```python
from build123d import *

# Parameters (mm, degrees)
SKETCH1_R           = 20.32
BOSS_EXTRUDE1_DEPTH = 26.0985
SKETCH2_W           = 14.0462
SKETCH2_H           = 14.0462
BOSS_EXTRUDE2_DEPTH = 7.7978
SKETCH3_R           = 4.953
BOSS_EXTRUDE3_DEPTH = 10.4013


with BuildPart() as part:
    # Sketch1 → Boss-Extrude1 (new body)
    with BuildSketch(Plane(origin=(0, 0, 0), x_dir=(1, 0, 0), z_dir=(0, 1, 0))):
        with Locations(Location((0, 0, 0), (0, 0, 270))):
            Circle(SKETCH1_R)
    extrude(amount=BOSS_EXTRUDE1_DEPTH)

    # Sketch2 → Boss-Extrude2 (add)
    with BuildSketch(Plane.XZ):
        Rectangle(SKETCH2_W, SKETCH2_H)
    extrude(amount=BOSS_EXTRUDE2_DEPTH)

    # Sketch3 → Boss-Extrude3 (add)
    with BuildSketch(Plane.XZ.offset(7.7978)):
        with Locations(Location((0, 0, 0), (0, 0, 90))):
            Circle(SKETCH3_R)
    extrude(amount=BOSS_EXTRUDE3_DEPTH)


solid = part.part
```
CAD build for the part. Positions are in the model's coordinates, mm. A direction names the side the tool comes from. Coordinates: 2 decimals unless noted, no trailing zeros. Order: outer loops, then holes, each group sorted by start corner. A loop starts at its lowest first (then second) coordinate and runs counter-clockwise, first axis right, second up. Notation, with made-up numbers: (-18, 5.5) -> (-1, 5.5) arc R26 cw to (-1, 28.5) -> close; hole circle Ø10 at (15, 69). An arc over 180 degrees is marked (long way). Use one line per item in the form item = value. Start each with the question number.
1) Drop flat-ended pins along their axis: pin 1 (5 mm diameter, centred on x = -15, z = 13, fed in from -Y); pin 2 (4 mm diameter, centred on y = -5.5, z = 2.5, fed in from -X); pin 3 (4 mm diameter, centred on y = -5, z = 0.5, fed in from +X). Give the stop position or say it passes through.
2) Band-saw the part on C-C on y = -12.5. Give the cut face in (x, z).
3) Band-saw the part on B-B on x = 0. Give the cut face in (y, z), then the cut area to 3 significant figures.
4) Tool access for faces 1 (the flat face through (7.023, -4, 0)), 2 (the cylindrical face through (-1.488, -12.926, 4.724)), 3 (the flat face through (0, -4, 7.023)): list every direction of +Z, -Z, +X, -X, +Y, -Y with a clear straight run to the whole face (end or side of a thin tool).
5) Band-saw the part on A-A on z = 0. Give the cut face in (x, y).
6) Drill centre lines: L1, parallel to Z at x = -0.5, y = 13.5; L2, parallel to Y at x = 8, z = 0. Where is each one in solid material? Low to high. Write a range as [from, to].
7) Band-saw the part on D-D on y = 18. Give the cut face in (x, z).
Entries:
q1.pin_1 = 0
q1.pin_2 = -7.02
q1.pin_3 = 7.02
q2.outline = circle Ø9.91 at (0, 0)
q3.outline = (-18.2, -4.95) -> (-7.8, -4.95) -> (-7.8, -7.02) -> (0, -7.02) -> (0, -20.32) -> (26.1, -20.32) -> (26.1, 20.32) -> (0, 20.32) -> (0, 7.02) -> (-7.8, 7.02) -> (-7.8, 4.95) -> (-18.2, 4.95) -> close
q3.area = 1,270 mm2
q4.face_1 = +Z, -Z, +X, -Y
q4.face_2 = -Y
q4.face_3 = +Z, +X, -X, -Y
q5.outline = (-20.32, 0) -> (-7.02, 0) -> (-7.02, -7.8) -> (-4.95, -7.8) -> (-4.95, -18.2) -> (4.95, -18.2) -> (4.95, -7.8) -> (7.02, -7.8) -> (7.02, 0) -> (20.32, 0) -> (20.32, 26.1) -> (-20.32, 26.1) -> close
q6.L1 = [-20.31, 20.31]
q6.L2 = [0, 26.1]
q7.outline = circle Ø40.64 at (0, 0)
